Could you check a few things on this model? Use its own coordinates, in mm. A direction names the side the tool comes from. Give positions to 0.01 mm unless a question says otherwise; leave off trailing zeros. Write each loop counter-clockwise with the first axis right and the second up, starting at its lowest first coordinate (ties: lowest second). Pieces come first, ordered by that corner, then holes. Notation, with made-up numbers: M 75,-25 L 106,-25 A25 ccw 106,8 Z; hole C 66,62 d8. An arc over 180 degrees is marked long. Answer as a JSON object with one key per item and string values. Group by question number.
Autodesk Inventor part; units mm, degrees
ref_plane "YZ Plane" through (0, 0, 0) normal (1, 0, 0) x (0, 1, 0)
ref_plane "XZ Plane" through (0, 0, 0) normal (0, 1, 0) x (-1, 0, 0)
ref_plane "XY Plane" through (0, 0, 0) normal (0, 0, 1) x (1, 0, 0)
sketch "Sketch1" plane through (0, 0, 0) normal (0, 0, 1) x (1, 0, 0)
  line L0 (0, 0) -> (10, 0)
  line L1 (10, 0) -> (12, 0)
  line L2 (10, 0) -> (10, 142.5)
  line L3 (0, 0) -> (0, 30)
  line L4 (12, 0) -> (12, 23.8)
  line L5 (12, 23.8) -> (12.5, 23.8)
  line L6 (12.5, 23.8) -> (12.5, 25.4)
  line L7 (12.5, 25.4) -> (12, 25.4)
  line L8 (12, 25.4) -> (12, 36.4)
  line L9 (12, 36.4) -> (12.5, 36.4)
  line L10 (12.5, 118.7) -> (12, 118.7)
  line L11 (12, 118.7) -> (12, 142.5)
  line L12 (12, 142.5) -> (10, 142.5)
  line L13 (12.5, 118.7) -> (12.5, 105.2)
  line L14 (12.5, 105.2) -> (12, 105.2)
  line L15 (12, 105.2) -> (12, 92.2)
  line L16 (12, 92.2) -> (12.5, 92.2)
  line L17 (12.5, 36.4) -> (12.5, 92.2)
  line L18 (12.5, 105.2) -> (12.5, 118.7)
  dimension "d0" = 10
  dimension "d1" = 2
  dimension "d2" = 142.5
  dimension "d4" = 30
  dimension "d6" = 23.8
  dimension "d7" = 0.5
  dimension "d8" = 1.6
  dimension "d9" = 11
  dimension "d10" = 90
  dimension "d11" = 0.5
  dimension "d12" = 82.3
  dimension "d13" = 13.5
  dimension "d14" = 0.5
  dimension "d15" = 13
revolve "Revolution1" add sketch "Sketch1" angle 360 about axis through (0, 0, 0) along (0, 1, 0)
properties part number "Axe manivelles"
1) I'm going to push flat-ended pins straight in: pin 1 (8 mm diameter, centred on x = -8, y = 72.5, fed in from +Z); pin 2 (4 mm diameter, centred on x = 7, y = 102, fed in from -Z); pin 3 (1 mm diameter, centred on y = 124, z = 2, fed in from -X). Where does each tip first touch, or does it pass through?
2) Please list where these lines run through material, in increasing order: line 1 along Z through (x, y) = (0, 30.5); line 2 along X through (y, z) = (46.5, 0). Write a range as from..to.
3) If we section it at C-C, the plane y = 113: List the corners of the cut face in (x, z) for me, plus the area to 3 significant figures.
4) We'd pull the mould along Z, two halves only. Please class faces 1 (the flat face through (-7, 23.8, -10)), 2 (the cylindrical face through (-2.17, 72.25, 9.76)), 3 (the cylindrical face through (-11.99, 98.61, 0.53)): released by +Z, released by -Z, zero draft, split by the parting line, or undercut.
5) For faces 4 (the cylindrical face through (11.923, 24.611, -3.755)), 5 (the flat face through (-7, 118.7, -10)), 6 (the flat face through (-7, 25.4, -10)), 7 (the cylindrical face through (-11.99, 12.07, -0.53)), which set-ups out of +Z, -Z, +X, -X, +Y, -Y let a thin tool reach every point of the face, with its end or its side?
Taken from the geometry:
{
 "1": {"pin 1": "z = 11.84", "pin 2": "z = -10.91", "pin 3": "x = -11.91"},
 "2": {"line 1": "-12..-10, 10..12", "line 2": "-12.5..-10, 10..12.5"},
 "3": {"outline": "C 0,0 d25; hole C 0,0 d20", "area": "177 mm²"},
 "4": {"face 1": "zero draft", "face 2": "undercut", "face 3": "split by the parting line"},
 "5": {"face 4": "+Y, -Y", "face 5": "+Y", "face 6": "none", "face 7": "-Y"}
}
